from build123d import *

# Parameters (mm, degrees)
F0_W     = 50
F0_H     = 50
F1_DEPTH = 75
F2_R     = 5
F3_DEPTH = 25
F4_R     = 5
F5_DEPTH = 25


with BuildPart() as f1:
    # F0 (on Top) → F1 (new body, symmetric)
    with BuildSketch(Plane.XY):
        Rectangle(F0_W, F0_H)
    extrude(amount=F1_DEPTH, both=True)

    # F2 (on face) → F3 (join)
    with BuildSketch(Plane(origin=(0, 0, -75), x_dir=(1, 0, 0), z_dir=(0, 0, -1))):
        Circle(F2_R)
    extrude(amount=F3_DEPTH)

    # F4 (on face) → F5 (join)
    with BuildSketch(Plane.XY.offset(75)):
        Circle(F4_R)
    extrude(amount=F5_DEPTH)


solid = f1.part
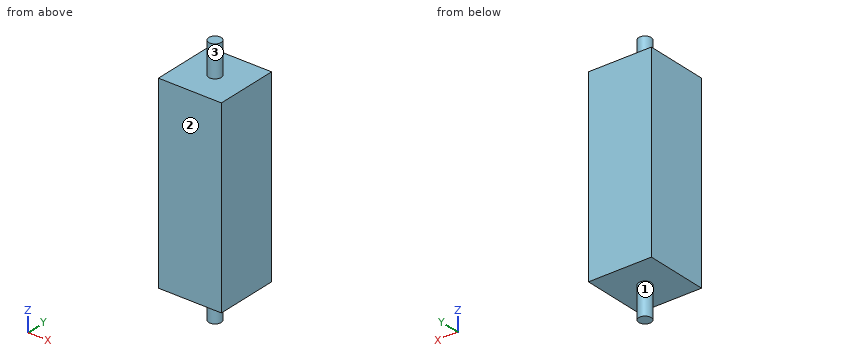
Work out the finished part from the listing and answer in its coordinate system (mm). Face numbers are marked on the shaded views. A direction names the side the tool comes from. Give positions to 0.01 mm unless a question says otherwise; leave off trailing zeros. Loops run counter-clockwise (first coordinate to the right, second up) from the corner with the lowest first, then second, coordinate; pieces in that order, holes last. Notation, with made-up numbers: (1.25, 63.5) - (11.25, 63.5) arc R27 cw to (11.25, 91.5) - close; hole circle Ø10 at (19, 41). An arc over 180 degrees is marked (long way). Answer in a Markdown table with one row per item. Add a question column.
Q1. The part is cut by section A-A (y = 0). Determine the outline of the cut face in (x, z), and give its area (3 significant figures).
Q2. The part is cut by section D-D (y = 18). Determine the outline of the cut face in (x, z), and give its area (3 significant figures).
Q3. Consider line 1 along Z through (x, y) = (-21, -22.5); line 2 along Y through (x, z) = (-0.5, 89). Determine where each line is inside the solid, lowest interval first.
Q4. This flat-tipped pin is pushed along its axis until it touches: P1, Ø8, axis at x = 19, y = -2, coming from the +Z side. Where does it stop, or does it pass through?
Q5. The part is cut by section C-C (z = -82). Determine the outline of the cut face in (x, y).
Q6. A tool of negligible diameter and unlimited length cuts with its end or side. For the marked faces 1, 2 and 3, from which of +Z, -Z, +X, -X, +Y, -Y can it reach the whole face along a straight path? Write none if from no direction.
Solution:
| question | item | result |
|---|---|---|
| 1 | outline | (-25, -75) - (-5, -75) - (-5, -100) - (5, -100) - (5, -75) - (25, -75) - (25, 75) - (5, 75) - (5, 100) - (-5, 100) - (-5, 75) - (-25, 75) - close |
| 1 | area | 8,000 mm² |
| 2 | outline | (-25, -75) - (25, -75) - (25, 75) - (-25, 75) - close |
| 2 | area | 7,500 mm² |
| 3 | line 1 | z = -75 to 75 |
| 3 | line 2 | y = -4.97 to 4.97 |
| 4 | P1 | stops at z = 75 |
| 5 | outline | circle Ø10 at (0, 0) |
| 6 | face 1 | -Z |
| 6 | face 2 | +Z, -Z, +X, -X, -Y |
| 6 | face 3 | +Z |
